Design review of the part built by this model. Coordinates are the model's own, in mm. A direction names the side the tool comes from. Round coordinates to 2 decimals unless told otherwise and drop trailing zeros. Order: outer loops, then holes, each group sorted by start corner. A loop starts at its lowest first (then second) coordinate and runs counter-clockwise, first axis right, second up. Notation, with made-up numbers: (29.5, 32.5) - (81.5, 32.5) arc R21 ccw to (81.5, 47.5) - close; hole circle Ø5 at (8, -35). An arc over 180 degrees is marked (long way). Write item = value, one per line.
from build123d import *
from build123d.topology import SkipClean

# Parameters (mm, degrees)
EXTRUDE_1_DEPTH     = 2
EXTRUDE_1_2_DEPTH   = 2
EXTRUDE_2_DEPTH     = 7
SKETCH_2_W          = 60.2
SKETCH_2_H          = 26.2
EXTRUDE_3_DEPTH     = 5.5
SKETCH_4_R          = 0.5
CUT_EXTRUDE_1_DEPTH = 0.5


with BuildPart() as part:
    # Sketch 1 → Extrude 1 (new body)
    with BuildSketch(Plane(origin=(0, 0, 0), x_dir=(1, 0, 0), z_dir=(0, 1, 0))):
        with BuildLine():
            Line((-32.1, -15.1), (32.1, -15.1))
            Line((32.1, -15.1), (32.1, 10.775))
            ThreePointArc((32.1, 10.775), (30.833236829, 13.833236829), (27.775, 15.1))
            Line((27.775, 15.1), (-27.775, 15.1))
            ThreePointArc((-27.775, 15.1), (-30.833236829, 13.833236829), (-32.1, 10.775))
            Line((-32.1, 10.775), (-32.1, -15.1))
        make_face()
        with BuildLine():
            Line((14.68883412, -12.6), (-14.68883412, -12.6))
            ThreePointArc((-14.68883412, -12.6), (-16.648480502, -10.999732483), (-15.472168434, -8.759786058))
            Line((-15.472168434, -8.759786058), (-0.783334313, -2.507106669))
            ThreePointArc((-0.783334313, -2.507106669), (0, -2.347320611), (0.783334313, -2.507106669))
            Line((0.783334313, -2.507106669), (15.472168434, -8.759786058))
            ThreePointArc((15.472168434, -8.759786058), (16.648480502, -10.999732483), (14.68883412, -12.6))
        make_face(mode=Mode.SUBTRACT)
        with BuildLine():
            Line((29.6, -7.401328038), (29.6, 7.401328038))
            ThreePointArc((29.6, 7.401328038), (28.703025696, 9.069660832), (26.816665687, 9.24154198))
            Line((26.816665687, 9.24154198), (9.429418868, 1.840213942))
            ThreePointArc((9.429418868, 1.840213942), (8.212753181, 0), (9.429418868, -1.840213942))
            Line((9.429418868, -1.840213942), (26.816665687, -9.24154198))
            ThreePointArc((26.816665687, -9.24154198), (28.703025696, -9.069660832), (29.6, -7.401328038))
        make_face(mode=Mode.SUBTRACT)
        with BuildLine():
            Line((14.68883412, 12.6), (-14.68883412, 12.6))
            ThreePointArc((-14.68883412, 12.6), (-16.648480502, 10.999732483), (-15.472168434, 8.759786058))
            Line((-15.472168434, 8.759786058), (-0.783334313, 2.507106669))
            ThreePointArc((-0.783334313, 2.507106669), (0, 2.347320611), (0.783334313, 2.507106669))
            Line((0.783334313, 2.507106669), (15.472168434, 8.759786058))
            ThreePointArc((15.472168434, 8.759786058), (16.648480502, 10.999732483), (14.68883412, 12.6))
        make_face(mode=Mode.SUBTRACT)
        with BuildLine():
            Line((-29.6, -7.401328038), (-29.6, 7.401328038))
            ThreePointArc((-29.6, 7.401328038), (-28.703025696, 9.069660832), (-26.816665687, 9.24154198))
            Line((-26.816665687, 9.24154198), (-9.429418868, 1.840213942))
            ThreePointArc((-9.429418868, 1.840213942), (-8.212753181, 0), (-9.429418868, -1.840213942))
            Line((-9.429418868, -1.840213942), (-26.816665687, -9.24154198))
            ThreePointArc((-26.816665687, -9.24154198), (-28.703025696, -9.069660832), (-29.6, -7.401328038))
        make_face(mode=Mode.SUBTRACT)
    extrude(amount=EXTRUDE_1_DEPTH)



with BuildPart() as body_2:
    # Sketch 1 → Extrude 1 2 (new body)
    with BuildSketch(Plane(origin=(0, 0, 0), x_dir=(1, 0, 0), z_dir=(0, 1, 0))):
        with BuildLine():
            Line((-27.775, -52.5), (27.775, -52.5))
            ThreePointArc((27.775, -52.5), (30.833236829, -51.233236829), (32.1, -48.175))
            Line((32.1, -48.175), (32.1, -22.3))
            Line((32.1, -22.3), (-32.1, -22.3))
            Line((-32.1, -22.3), (-32.1, -48.175))
            ThreePointArc((-32.1, -48.175), (-30.833236829, -51.233236829), (-27.775, -52.5))
        make_face()
        with BuildLine():
            Line((-0.783334313, -34.892893331), (-15.472168434, -28.640213942))
            ThreePointArc((-15.472168434, -28.640213942), (-16.648480502, -26.400267517), (-14.68883412, -24.8))
            Line((-14.68883412, -24.8), (14.68883412, -24.8))
            ThreePointArc((14.68883412, -24.8), (16.648480502, -26.400267517), (15.472168434, -28.640213942))
            Line((15.472168434, -28.640213942), (0.783334313, -34.892893331))
            ThreePointArc((0.783334313, -34.892893331), (0, -35.052679389), (-0.783334313, -34.892893331))
        make_face(mode=Mode.SUBTRACT)
        with BuildLine():
            Line((-9.429418868, -39.240213942), (-26.816665687, -46.64154198))
            ThreePointArc((-26.816665687, -46.64154198), (-28.703025696, -46.469660832), (-29.6, -44.801328038))
            Line((-29.6, -44.801328038), (-29.6, -29.998671962))
            ThreePointArc((-29.6, -29.998671962), (-28.703025696, -28.330339168), (-26.816665687, -28.15845802))
            Line((-26.816665687, -28.15845802), (-9.429418868, -35.559786058))
            ThreePointArc((-9.429418868, -35.559786058), (-8.212753181, -37.4), (-9.429418868, -39.240213942))
        make_face(mode=Mode.SUBTRACT)
        with BuildLine():
            Line((0.783334313, -39.907106669), (15.472168434, -46.159786058))
            ThreePointArc((15.472168434, -46.159786058), (16.648480502, -48.399732483), (14.68883412, -50))
            Line((14.68883412, -50), (-14.68883412, -50))
            ThreePointArc((-14.68883412, -50), (-16.648480502, -48.399732483), (-15.472168434, -46.159786058))
            Line((-15.472168434, -46.159786058), (-0.783334313, -39.907106669))
            ThreePointArc((-0.783334313, -39.907106669), (0, -39.747320611), (0.783334313, -39.907106669))
        make_face(mode=Mode.SUBTRACT)
        with BuildLine():
            Line((29.6, -44.801328038), (29.6, -29.998671962))
            ThreePointArc((29.6, -29.998671962), (28.703025696, -28.330339168), (26.816665687, -28.15845802))
            Line((26.816665687, -28.15845802), (9.429418868, -35.559786058))
            ThreePointArc((9.429418868, -35.559786058), (8.212753181, -37.4), (9.429418868, -39.240213942))
            Line((9.429418868, -39.240213942), (26.816665687, -46.64154198))
            ThreePointArc((26.816665687, -46.64154198), (28.703025696, -46.469660832), (29.6, -44.801328038))
        make_face(mode=Mode.SUBTRACT)
    extrude(amount=EXTRUDE_1_2_DEPTH)


with BuildPart() as part_1:
    with SkipClean():  # the faces are left unmerged after this step: merging them gives an invalid solid
        add(part.part)

        add(body_2.part)  # Extrude 2 merges body 2
        # Sketch 3 → Extrude 2 (add)
        with BuildSketch(Plane(origin=(0, 0, 0), x_dir=(1, 0, 0), z_dir=(0, 1, 0))):
            with BuildLine():
                Line((-32.1, -15.1), (-32.1, 10.775))
                ThreePointArc((-32.1, 10.775), (-30.833236829, 13.833236829), (-27.775, 15.1))
                Line((-27.775, 15.1), (27.775, 15.1))
                ThreePointArc((27.775, 15.1), (30.833236829, 13.833236829), (32.1, 10.775))
                Line((32.1, 10.775), (32.1, -15.1))
                Line((32.1, -15.1), (32.1, -22.3))
                Line((32.1, -22.3), (32.1, -48.175))
                ThreePointArc((32.1, -48.175), (30.833236829, -51.233236829), (27.775, -52.5))
                Line((27.775, -52.5), (-27.775, -52.5))
                ThreePointArc((-27.775, -52.5), (-30.833236829, -51.233236829), (-32.1, -48.175))
                Line((-32.1, -48.175), (-32.1, -22.3))
                Line((-32.1, -22.3), (-32.1, -15.1))
            make_face()
            with BuildLine():
                Line((-30.1, -17.425), (-30.1, -19.975))
                ThreePointArc((-30.1, -19.975), (-29.419023266, -21.619023266), (-27.775, -22.3))
                Line((-27.775, -22.3), (27.775, -22.3))
                ThreePointArc((27.775, -22.3), (29.419023266, -21.619023266), (30.1, -19.975))
                Line((30.1, -19.975), (30.1, -17.425))
                ThreePointArc((30.1, -17.425), (29.419023266, -15.780976734), (27.775, -15.1))
                Line((27.775, -15.1), (-27.775, -15.1))
                ThreePointArc((-27.775, -15.1), (-29.419023266, -15.780976734), (-30.1, -17.425))
            make_face(mode=Mode.SUBTRACT)
            with BuildLine():
                Line((-27.775, -13.1), (27.775, -13.1))
                ThreePointArc((27.775, -13.1), (29.419023266, -12.419023266), (30.1, -10.775))
                Line((30.1, -10.775), (30.1, 10.775))
                ThreePointArc((30.1, 10.775), (29.419023266, 12.419023266), (27.775, 13.1))
                Line((27.775, 13.1), (-27.775, 13.1))
                ThreePointArc((-27.775, 13.1), (-29.419023266, 12.419023266), (-30.1, 10.775))
                Line((-30.1, 10.775), (-30.1, -10.775))
                ThreePointArc((-30.1, -10.775), (-29.419023266, -12.419023266), (-27.775, -13.1))
            make_face(mode=Mode.SUBTRACT)
            with BuildLine():
                Line((-30.1, -48.175), (-30.1, -26.625))
                ThreePointArc((-30.1, -26.625), (-29.419023266, -24.980976734), (-27.775, -24.3))
                Line((-27.775, -24.3), (27.775, -24.3))
                ThreePointArc((27.775, -24.3), (29.419023266, -24.980976734), (30.1, -26.625))
                Line((30.1, -26.625), (30.1, -48.175))
                ThreePointArc((30.1, -48.175), (29.419023266, -49.819023266), (27.775, -50.5))
                Line((27.775, -50.5), (-27.775, -50.5))
                ThreePointArc((-27.775, -50.5), (-29.419023266, -49.819023266), (-30.1, -48.175))
            make_face(mode=Mode.SUBTRACT)
        extrude(amount=EXTRUDE_2_DEPTH)
    add(part_1.part.scale(1), mode=Mode.REPLACE)  # the faces are merged on a copy

    # Sketch 2 → Extrude 3 (add)
    # profile 1 of 2: a face of its own
    with BuildSketch(Plane(origin=(0, 0, 0), x_dir=(1, 0, 0), z_dir=(0, 1, 0))):
        Rectangle(SKETCH_2_W, SKETCH_2_H)
        with BuildLine():
            Line((27.775, -12.6), (-27.775, -12.6))
            ThreePointArc((-27.775, -12.6), (-29.065469876, -12.065469876), (-29.6, -10.775))
            Line((-29.6, -10.775), (-29.6, 10.775))
            ThreePointArc((-29.6, 10.775), (-29.065469876, 12.065469876), (-27.775, 12.6))
            Line((-27.775, 12.6), (27.775, 12.6))
            ThreePointArc((27.775, 12.6), (29.065469876, 12.065469876), (29.6, 10.775))
            Line((29.6, 10.775), (29.6, -10.775))
            ThreePointArc((29.6, -10.775), (29.065469876, -12.065469876), (27.775, -12.6))
        make_face(mode=Mode.SUBTRACT)
    # profile 2 of 2: a face of its own
    with BuildSketch(Plane(origin=(0, 0, 0), x_dir=(1, 0, 0), z_dir=(0, 1, 0))):
        with Locations((0, -37.4)):
            Rectangle(SKETCH_2_W, SKETCH_2_H)
        with BuildLine():
            Line((27.775, -24.8), (-27.775, -24.8))
            ThreePointArc((-27.775, -24.8), (-29.065469876, -25.334530124), (-29.6, -26.625))
            Line((-29.6, -26.625), (-29.6, -48.175))
            ThreePointArc((-29.6, -48.175), (-29.065469876, -49.465469876), (-27.775, -50))
            Line((-27.775, -50), (27.775, -50))
            ThreePointArc((27.775, -50), (29.065469876, -49.465469876), (29.6, -48.175))
            Line((29.6, -48.175), (29.6, -26.625))
            ThreePointArc((29.6, -26.625), (29.065469876, -25.334530124), (27.775, -24.8))
        make_face(mode=Mode.SUBTRACT)
    extrude(amount=EXTRUDE_3_DEPTH)

    # Sketch 4 → Cut-Extrude 1 (cut)
    with BuildSketch(Plane.XZ):
        with Locations(Location((-30.85, 42.3, 0), (0, 0, 270))):
            Circle(SKETCH_4_R)
        with Locations(Location((3.95, 37.4, 0), (0, 0, 270))):
            Circle(SKETCH_4_R)
        with Locations(Location((31.3, 36.2, 0), (0, 0, 270))):
            Circle(SKETCH_4_R)
        with Locations(Location((31.3, 1.2, 0), (0, 0, 270))):
            Circle(SKETCH_4_R)
        with Locations(Location((3.95, 0, 0), (0, 0, 270))):
            Circle(SKETCH_4_R)
        with Locations(Location((-30.85, -4.9, 0), (0, 0, 270))):
            Circle(SKETCH_4_R)
    extrude(amount=-CUT_EXTRUDE_1_DEPTH, mode=Mode.SUBTRACT)


solid = part_1.part
Item 1: For line 1 along Z through (x, y) = (9, 4.75); line 2 along X through (y, z) = (0.15, 37.4); line 3 along X through (y, z) = (6.5, 31.5), list the stretches that pass through material, from the lowest coordinate up. Write a range as [from, to].
Data:
line_1 = [-15.1, -12.6], [12.6, 15.1], [22.3, 24.8], [50, 52.5]
line_2 = [-32.1, -29.6], [-8.21, 3.45], [4.45, 8.21], [29.6, 32.1]
line_3 = [-32.1, -30.1], [30.1, 32.1]
Item 2: Take a section at B-B, the plane z = 5.5. State the section outline as (x, y) points, and give its area (3 significant figures).
Data:
outline = (-32.1, 0) - (-29.6, 0) - (-29.6, 5.5) - (-30.1, 5.5) - (-30.1, 7) - (-32.1, 7) - close; (-18.03, 0) - (-7.81, 0) - (-7.81, 2) - (-18.03, 2) - close; (7.81, 0) - (18.03, 0) - (18.03, 2) - (7.81, 2) - close; (29.6, 0) - (32.1, 0) - (32.1, 7) - (30.1, 7) - (30.1, 5.5) - (29.6, 5.5) - close
area = 74.4 mm2
Item 3: The part is to be moulded in two halves that separate along Z. For faces 3 (the face through (-30.799, 3.451, 51.267)), 4 (the face through (-29.05, 3.73, 12.08)), say which applies: +Z half, -Z half, draft (parallel to the pull), parting line (faces both ways), or undercut.
Data:
face_3 = +Z half
face_4 = undercut
Item 4: For faces 1 (the face through (29.44, 3.45, 15.8)), 2 (the face through (29.4, 6.24, 12.44)), list the 3-axis set-ups (+Z, -Z, +X, -X, +Y, -Y) from which the entire face can be reached by the end or side of a thin tool; tool diameter is ignored.
Data:
face_1 = +Y, -Y
face_2 = +Y
Item 5: Insertion check: P1, Ø7.5, axis at x = 1, z = 38, coming from the +Y side. The pin has a flat end and moves straight along its axis. Give the tip position at first contact, or say it passes through.
Data:
P1 = 2
Item 6: Take a section at A-A, the plane y = 6.25. Count the separate pieces of the cut face and the enclosed holes in it, and give its area (3 significant figures).
Data:
separate_pieces = 1
enclosed_holes = 3
area = 750 mm2
